Check sheet for the modelled part. Datum: model origin and axes. Units: mm. A direction names the side the tool comes from. Round coordinates to 2 decimals unless told otherwise and drop trailing zeros. Write each loop counter-clockwise with the first axis right and the second up, starting at its lowest first coordinate (ties: lowest second). Pieces come first, ordered by that corner, then holes.
Item 1: Section check C-C, the plane y = -73. Record the cut outline in (x, z), plus the area to 3 significant figures.
Item 2: Section check B-B, the plane x = 7. Record the cut outline in (y, z).
Item 3: Material ranges on line 1 along Y through (x, z) = (24, 10.5); line 2 along Z through (x, y) = (52.5, -63), recorded low to high.
Item 4: Depth check by flat-ended pin: pin 1 (0.8 mm diameter, centred on x = 96.5, z = 11, fed in from +Y); pin 2 (1 mm diameter, centred on x = -4.5, y = -69.5, fed in from +Z); pin 3 (12 mm diameter, centred on x = 30.5, z = 22, fed in from -Y); pin 4 (10 mm diameter, centred on y = -49, z = 19.5, fed in from +X). Enter the tip coordinate at first touch or a pass-through.
Item 5: Set-up check for faces 1 (the flat face through (26, -47, 10)), 2 (the flat face through (26, 7, 30)): record each of +Z, -Z, +X, -X, +Y, -Y from which the full face is reachable in a straight line by a thin tool's end or side.
Item 6: Section check A-A, the plane z = 26. Record the cut outline in (x, y).
from build123d import *

# Parameters (mm, degrees)
ESQUISSE1_W             = 160
ESQUISSE1_H             = 108
BOSS_EXTRU_1_DEPTH      = 10
ESQUISSE2_W             = 160
ESQUISSE2_H             = 30
BOSS_EXTRU_2_DEPTH      = 20
ESQUISSE3_W             = 1
ESQUISSE3_H             = 30
ENL_V_MAT_EXTRU_1_DEPTH = 1


with BuildPart() as part:
    # Esquisse1 → Boss.-Extru.1 (new body)
    with BuildSketch(Plane.XY):
        with Locations((27.187647666, -32.051659751)):
            Rectangle(ESQUISSE1_W, ESQUISSE1_H)
    extrude(amount=BOSS_EXTRU_1_DEPTH)

    # Esquisse2 → Boss.-Extru.2 (add)
    with BuildSketch(Plane.XY.offset(10)):
        with Locations((27.187647666, 6.948340249)):
            Rectangle(ESQUISSE2_W, ESQUISSE2_H)
    extrude(amount=BOSS_EXTRU_2_DEPTH)

    # Esquisse3 → Enlèv. mat.-Extru.1 (cut)
    with BuildSketch(Plane(origin=(0, 21.948340249, 0), x_dir=(1, 0, 0), z_dir=(0, 1, 0))):
        with Locations((96.687647666, -15)):
            Rectangle(ESQUISSE3_W, ESQUISSE3_H)
    extrude(amount=-ENL_V_MAT_EXTRU_1_DEPTH, mode=Mode.SUBTRACT)


solid = part.part
Values found:
1. outline: (-52.81, 0) - (107.19, 0) - (107.19, 10) - (-52.81, 10) - close
1. area: 1,600 mm2
2. outline: (-86.05, 0) - (21.95, 0) - (21.95, 30) - (-8.05, 30) - (-8.05, 10) - (-86.05, 10) - close
3. line 1: y = -8.05 to 21.95
3. line 2: z = 0 to 10
4. pin 1: stops at y = 21.95
4. pin 2: stops at z = 10
4. pin 3: stops at y = -8.05
4. pin 4: passes through
5. face 1: +Z, +X, -X, -Y
5. face 2: +Z, +X, -X, +Y, -Y
6. outline: (-52.81, -8.05) - (107.19, -8.05) - (107.19, 21.95) - (97.19, 21.95) - (97.19, 20.95) - (96.19, 20.95) - (96.19, 21.95) - (-52.81, 21.95) - close
